Source: three-view drawing plus pictorial views. Frame: mm from the lowest corner of the part. A direction names the side the tool comes from. Give positions to 0.01 mm unless a question says otherwise; leave off trailing zeros. Loops run counter-clockwise (first coordinate to the right, second up) from the corner with the lowest first, then second, coordinate; pieces in that order, holes last. Notation, with made-up numbers: M 89,-25.5 L 98,-25.5 A34 ccw 98,5.5 Z; hole C -14.75,8.25 d9. An arc over 180 degrees is marked long. Answer as a JSON object with one key per item and string values. Group by question number.
1) Draft query along X for the marked faces 3, 4, 5 and 6. Return one class per face: +X half, -X half, draft (parallel to the pull), parting line (faces both ways), or undercut.
2) Ray query, L1, parallel to X at y = 2.15, z = 32; L2, parallel to X at y = 24.5, z = 35; L3, parallel to Y at x = 20, z = 42. Return the intervals inside material, ascending.
3) Section query A-A on z = 8. Return loops of the section in (x, y), plus the area to 3 significant figures.
4) Access query for the marked faces 1 and 2. Directions: +Z, -Z, +X, -X, +Y, -Y. A direction counts if a zero-diameter tool reaches every point of the face in a straight line with its end or side. Return the directions, or none.
5) First-contact query: P1, Ø2, axis at x = 8, z = 33, coming from the +Y side. Flat tip, straight axial feed; report the tip coordinate or a pass-through.
6) Section query D-D on x = 20. Return loops of the section in (y, z), plus the area to 3 significant figures.
7) Section query C-C on y = 26. Return loops of the section in (x, z), plus the area to 3 significant figures.
8) Section query B-B on x = 7.5. Return loops of the section in (y, z), plus the area to 3 significant figures.
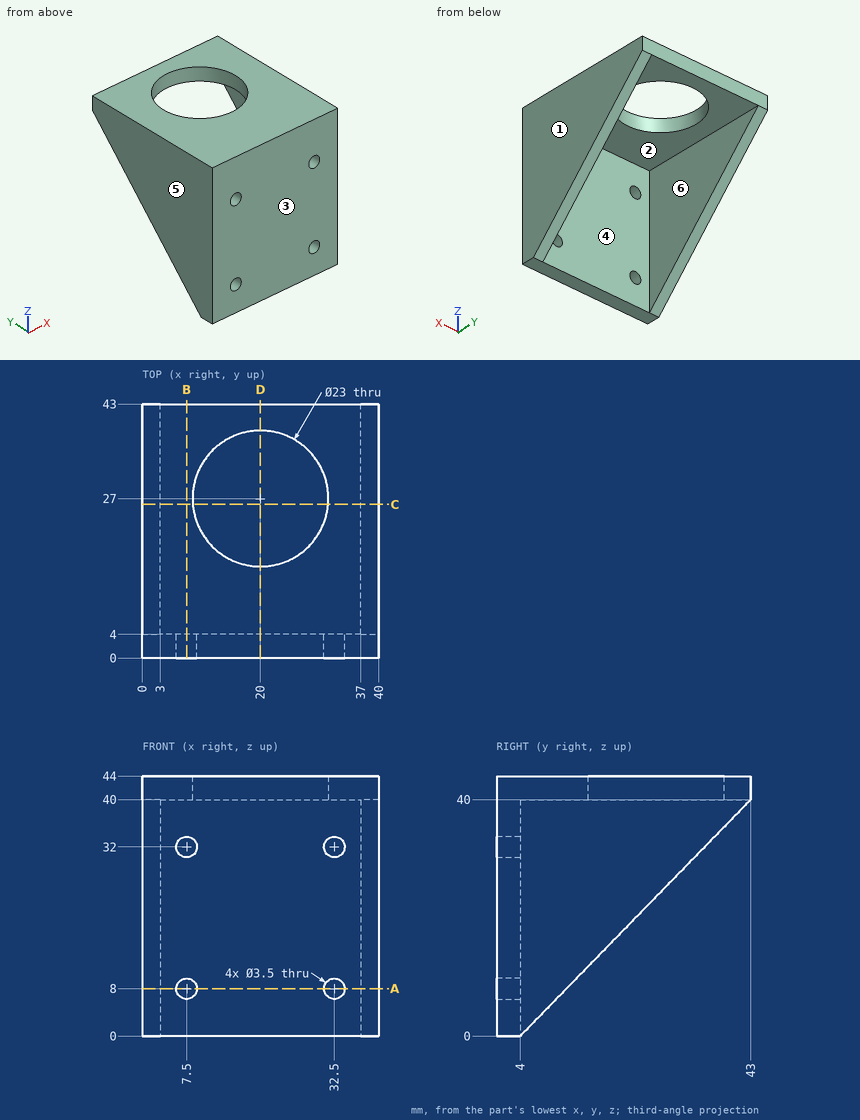
Output:
{
 "1": {"face 3": "draft", "face 4": "undercut", "face 5": "-X half", "face 6": "undercut"},
 "2": {"L1": "x = 0 to 5.75, 9.25 to 30.75, 34.25 to 40", "L2": "x = 0 to 3, 37 to 40", "L3": "y = 0 to 15.5, 38.5 to 43"},
 "3": {"outline": "M 0,0 L 5.75,0 L 5.75,4 L 3,4 L 3,11.8 L 0,11.8 Z; M 9.25,0 L 30.75,0 L 30.75,4 L 9.25,4 Z; M 34.25,0 L 40,0 L 40,11.8 L 37,11.8 L 37,4 L 34.25,4 Z", "area": "179 mm^2"},
 "4": {"face 1": "+Z, -Z, +X, +Y, -Y", "face 2": "-Z, +Y"},
 "5": {"P1": "stops at y = 4"},
 "6": {"outline": "M 0,0 L 4,0 L 4,40 L 15.5,40 L 15.5,44 L 0,44 Z; M 38.5,40 L 43,40 L 43,44 L 38.5,44 Z", "area": "240 mm^2"},
 "7": {"outline": "M 0,22.56 L 3,22.56 L 3,40 L 8.54,40 L 8.54,44 L 0,44 Z; M 31.46,40 L 37,40 L 37,22.56 L 40,22.56 L 40,44 L 31.46,44 Z", "area": "173 mm^2"},
 "8": {"outline": "M 0,0 L 4,0 L 4,6.25 L 0,6.25 Z; M 0,9.75 L 4,9.75 L 4,30.25 L 0,30.25 Z; M 0,33.75 L 4,33.75 L 4,40 L 43,40 L 43,44 L 0,44 Z", "area": "304 mm^2"}
}
